```python
from build123d import *

# Parameters (mm, degrees)
EXTRUDE_1_DEPTH     = 81
SHELL_1_T           = -2
FILLET_1_R          = 4
FILLET_2_R          = 2
CUT_EXTRUDE_START   = -76.5
CUT_EXTRUDE_1_DEPTH = 76.5
EXTRUDE_2_DEPTH     = 4
EXTRUDE_3_DEPTH     = 2
FILLET_3_R          = 1
FILLET_4_R          = 0.5


with BuildPart() as part:
    # 草图1 → 凸台-拉伸1 (new body)
    with BuildSketch(Plane.XY):
        with BuildLine():
            Line((0, 0), (8, 0))
            Line((8, 0), (22, 0))
            ThreePointArc((22, 0), (17.899494937, 9.899494937), (8, 14))
            Line((8, 14), (-8, 14))
            ThreePointArc((-8, 14), (-17.899494937, 9.899494937), (-22, 0))
            Line((-22, 0), (-8, 0))
            Line((-8, 0), (0, 0))
        make_face()
    extrude(amount=-EXTRUDE_1_DEPTH)

    # 抽壳1
    shell_1_openings = [part.faces().sort_by_distance(p)[0] for p in [
        (0, 6.387452756, -81),
        (0, 0, -40.5),
    ]]
    offset(amount=SHELL_1_T, openings=shell_1_openings, kind=Kind.INTERSECTION)

    # 圆角1
    fillet_1_edges = [part.edges().sort_by_distance(p)[0] for p in [
        (-17.899494937, 9.899494937, 0),
        (0, 14, 0),
        (17.899494937, 9.899494937, 0),
    ]]
    fillet(fillet_1_edges, radius=FILLET_1_R)

    # 圆角2
    fillet_2_edges = [part.edges().sort_by_distance(p)[0] for p in [
        (16.485281374, 8.485281374, -2),
        (0, 12, -2),
        (-16.485281374, 8.485281374, -2),
    ]]
    fillet(fillet_2_edges, radius=FILLET_2_R)

    # 草图2 → 切除-拉伸1 (cut)
    with BuildSketch(Plane(origin=(0, 0, -81), x_dir=(-1, 0, 0), z_dir=(0, 0, -1)).offset(CUT_EXTRUDE_START)):
        with BuildLine():
            Line((-20, 0), (-21.05, 0))
            Line((-21.05, 0), (-20.992430448, 1.098492488))
            Line((-20.992430448, 1.098492488), (-19.949615653, 1.098492488))
            ThreePointArc((-19.949615653, 1.098492488), (-19.987397295, 0.549823683), (-20, 0))
        make_face()
        with BuildLine():
            Line((20, 0), (21.05, 0))
            Line((21.05, 0), (20.992430448, 1.098492488))
            Line((20.992430448, 1.098492488), (19.949615653, 1.098492488))
            ThreePointArc((19.949615653, 1.098492488), (19.987397295, 0.549823683), (20, 0))
        make_face()
    extrude(amount=CUT_EXTRUDE_1_DEPTH, mode=Mode.SUBTRACT)

    # 草图3 → 凸台-拉伸2 (add, symmetric)
    with BuildSketch(Plane(origin=(0, 0, 0), x_dir=(0, 0, -1), z_dir=(1, 0, 0))):
        Polygon((81, 12), (81, 13), (78, 13), (78, 10.5), (81, 10.5), (86, 10.5), (86, 12), (84.5, 13), (83.5, 13), (83.5, 12), align=None)
    extrude(amount=EXTRUDE_2_DEPTH, both=True)

    # 草图4 → 凸台-拉伸3 (add)
    with BuildSketch(Plane.XY):
        Polygon((-8, 0), (-6, 0), (-3, -3), (-6, -3), (-10, -3), (-13, -3), (-10, 0), align=None)
        Polygon((3, -3), (6, 0), (8, 0), (10, 0), (13, -3), (10, -3), (6, -3), align=None)
    extrude(amount=-EXTRUDE_3_DEPTH)

    # 圆角3
    fillet_3_edges = [part.edges().sort_by_distance(p)[0] for p in [
        (-3, -3, -1),
        (-13, -3, -1),
        (3, -3, -1),
        (13, -3, -1),
    ]]
    fillet(fillet_3_edges, radius=FILLET_3_R)

    # 圆角4
    fillet_4_edges = [part.edges().sort_by_distance(p)[0] for p in [
        (-10, 0, -1),
        (-6, 0, -1),
        (6, 0, -1),
        (10, 0, -1),
    ]]
    fillet(fillet_4_edges, radius=FILLET_4_R)


solid = part.part
```
Could you check a few things on this model? Use its own coordinates, in mm. A direction names the side the tool comes from. Round coordinates to 2 decimals unless told otherwise and drop trailing zeros. Loops run counter-clockwise (first coordinate to the right, second up) from the corner with the lowest first, then second, coordinate; pieces in that order, holes last. Notation, with made-up numbers: (63.5, 11.5) -> (122.5, 11.5) arc R22 cw to (122.5, 18.5) -> close; hole circle Ø10 at (77.5, 73.5). An arc over 180 degrees is marked (long way). Put each result on its own line as item: value.
Q1. I want a section at A-A on z = -63. Write out the boundary of the cut face in (x, y).
Checks:
outline: (-22, 0) -> (-21.05, 0) -> (-20.99, 1.1) -> (-19.95, 1.1) arc R12 cw to (-8, 12) -> (8, 12) arc R12 cw to (19.95, 1.1) -> (20.99, 1.1) -> (21.05, 0) -> (22, 0) arc R14 ccw to (8, 14) -> (-8, 14) arc R14 ccw to start
Q2. For pin 1 Ø5 at (x, z) = (3, -63) entering from -Y; pin 2 Ø3 at (y, z) = (11, -60) entering from -X; pin 3 Ø1.6 at (x, y) = (0.5, 11.5) entering from +Z, each with a flat end and sliding along its axis, tell me the tip position at first contact or that it passes through.
Checks:
pin 1: y = 12
pin 2: x = -18.28
pin 3: z = -0.06
Q3. Please list where these lines run through material, in increasing order: line 1 (X direction, y = 0.25, z = -71); line 2 (Z direction, x = -18, y = 1.5); line 3 (Y direction, x = -8.5, z = -45). Write a range as from..to.
Checks:
line 1: -22..-21.04, 21.04..22
line 2: -2..0
line 3: 11.99..13.99
Q4. Thinking about a two-plate mould opening in Y: for faces 4 (the cylindrical face through (-4.497, -2.398, -1.014)), 5 (the flat face through (0.056, 12.493, -85.26)), 6 (the flat face through (0, 4, 0)), which applies, pulls with the +Y half, pulls with the -Y half, needs draft (parallel to the pull), parting line crosses it, or undercut?
Checks:
face 4: undercut
face 5: pulls with the +Y half
face 6: needs draft
Q5. Which directions (+Z, -Z, +X, -X, +Y, -Y) give clear straight access to the entire face, cutting with the end or side of a thin tool? Please do faces 1 (the flat face through (8, -3, -1)), 2 (the cylindrical face through (16.58, 8.39, -41.96)), 3 (the flat face through (0, 12, -82)).
Checks:
face 1: +Z, -Z, +X, -X, -Y
face 2: -Z, -Y
face 3: +X, -X, +Y
